Geometry: final body of the model. Coordinates: model frame, mm. A direction names the side the tool comes from. Give positions to 0.01 mm unless a question says otherwise; leave off trailing zeros. Write each loop counter-clockwise with the first axis right and the second up, starting at its lowest first coordinate (ties: lowest second). Pieces come first, ordered by that corner, then holes. Notation, with made-up numbers: (25, -31) -> (79, -31) arc R28 ccw to (79, 1) -> close; hole circle Ø6 at (-37, -36). An arc over 180 degrees is marked (long way). Answer as a JSON object with one key per item and string values. Group by question number.
(1) Contact query for flat-ended pins moving along their axis: pin 1 Ø6.5 at (x, z) = (0, 0) entering from +Y; pin 2 Ø1 at (y, z) = (3, 0) entering from +X; pin 3 Ø1 at (x, z) = (-6.5, 1) entering from +Y. Output: stop coordinate, or through.
(2) Section query A-A on z = 0. Output: boundary loops of the cut face in (x, y), plus the area to 3 significant figures.
(3) Section query D-D on z = 6. Output: boundary loops of the cut face in (x, y), plus the area to 3 significant figures.
(4) Section query C-C on y = 3.3. Output: boundary loops of the cut face in (x, z), plus the area to 3 significant figures.
(5) Draft query along X for faces 3 (the face through (5, 2, 2)), 4 (the face through (-1, 1, 2)), 5 (the face through (-9.76, 0.99, -2.17)). Return one class per face: +X half, -X half, draft (parallel to the pull), parting line (faces both ways), or undercut.
(6) Material intervals for probe 1 along X at (y, z) = (1.6, 0); probe 2 along X at (y, z) = (0.3, 0); probe 3 along Y at (x, z) = (1.5, 3.5), sorted ascending.
(7) Section query B-B on x = 0. Output: boundary loops of the cut face in (y, z).
(8) Set-up query: faces 1 (the face through (0, 0, 2)), 2 (the face through (-3.905, 2.521, -0.867)). Return all of +Z, -Z, +X, -X, +Y, -Y with unobstructed straight access to the full face (end or side cutting, diameter ignored); none if empty.
from build123d import *

# Parameters (mm, degrees)
SKETCH_1_R          = 10
EXTRUDE_1_DEPTH     = 2
SKETCH_2_R          = 5
EXTRUDE_2_DEPTH     = 2
SKETCH_3_R          = 1.75
CUT_EXTRUDE_1_DEPTH = 15.696938457
SKETCH_4_R          = 4
CUT_EXTRUDE_2_DEPTH = 3


with BuildPart() as part:
    # 草图1 → 凸台-拉伸1 (new body)
    with BuildSketch(Plane(origin=(0, 0, 0), x_dir=(1, 0, 0), z_dir=(0, 1, 0))):
        with Locations(Location((0, 0, 0), (0, 0, 270))):
            Circle(SKETCH_1_R)
    extrude(amount=EXTRUDE_1_DEPTH)

    # 草图2 → 凸台-拉伸2 (add)
    with BuildSketch(Plane(origin=(0, 2, 0), x_dir=(1, 0, 0), z_dir=(0, 1, 0))):
        with Locations(Location((0, 0, 0), (0, 0, 270))):
            Circle(SKETCH_2_R)
    extrude(amount=EXTRUDE_2_DEPTH)

    # 草图3 → 切除-拉伸1 (cut, through all)
    with BuildSketch(Plane(origin=(0, 4, 0), x_dir=(1, 0, 0), z_dir=(0, 1, 0))):
        with Locations(Location((0, 0, 0), (0, 0, 270))):
            Circle(SKETCH_3_R)
    extrude(amount=-CUT_EXTRUDE_1_DEPTH, mode=Mode.SUBTRACT)

    # 草图4 → 切除-拉伸2 (cut)
    with BuildSketch(Plane(origin=(0, 4, 0), x_dir=(1, 0, 0), z_dir=(0, 1, 0))):
        with Locations(Location((0, 0, 0), (0, 0, 270))):
            Circle(SKETCH_4_R)
    extrude(amount=-CUT_EXTRUDE_2_DEPTH, mode=Mode.SUBTRACT)


solid = part.part
Answer list:
{
 "1": {"pin 1": "y = 1", "pin 2": "x = 5", "pin 3": "y = 2"},
 "2": {"outline": "(-10, 0) -> (-1.75, 0) -> (-1.75, 1) -> (-4, 1) -> (-4, 4) -> (-5, 4) -> (-5, 2) -> (-10, 2) -> close; (1.75, 0) -> (10, 0) -> (10, 2) -> (5, 2) -> (5, 4) -> (4, 4) -> (4, 1) -> (1.75, 1) -> close", "area": "32.5 mm2"},
 "3": {"outline": "(-8, 0) -> (8, 0) -> (8, 2) -> (-8, 2) -> close", "area": "32.0 mm2"},
 "4": {"outline": "circle Ø10 at (0, 0); hole circle Ø8 at (0, 0)", "area": "28.3 mm2"},
 "5": {"face 3": "draft", "face 4": "undercut", "face 5": "parting line"},
 "6": {"probe 1": "-10 to -4, 4 to 10", "probe 2": "-10 to -1.75, 1.75 to 10", "probe 3": "0 to 1"},
 "7": {"outline": "(0, -10) -> (2, -10) -> (2, -5) -> (4, -5) -> (4, -4) -> (1, -4) -> (1, -1.75) -> (0, -1.75) -> close; (0, 1.75) -> (1, 1.75) -> (1, 4) -> (4, 4) -> (4, 5) -> (2, 5) -> (2, 10) -> (0, 10) -> close"},
 "8": {"face 1": "+Z, -Z, +X, -X, -Y", "face 2": "+Y"}
}
